CAD build for the part. Positions are in the model's coordinates, mm. A direction names the side the tool comes from. Round coordinates to 2 decimals unless told otherwise and drop trailing zeros. Loops run counter-clockwise (first coordinate to the right, second up) from the corner with the lowest first, then second, coordinate; pieces in that order, holes last.
from build123d import *

# Parameters (mm, degrees)
SKETCH_1_R          = 30
SKETCH_1_R_2        = 1.6
SKETCH_1_R_3        = 13.5
EXTRUDE_1_DEPTH     = 6
SKETCH_2_W          = 8
SKETCH_2_H          = 40
EXTRUDE_2_DEPTH     = 6
SKETCH_3_R          = 1.6
CUT_EXTRUDE_1_DEPTH = 6
SKETCH_4_R          = 3.25
CUT_EXTRUDE_2_DEPTH = 3


with BuildPart() as part:
    # 草图1 → 凸台-拉伸1 (new body)
    with BuildSketch(Plane(origin=(0, 0, 0), x_dir=(1, 0, 0), z_dir=(0, 1, 0))):
        with Locations(Location((15, 90, 0), (0, 0, 270))):
            Circle(SKETCH_1_R)
        with Locations(Location((30.5, 105.5, 0), (0, 0, 270))):
            Circle(SKETCH_1_R_2, mode=Mode.SUBTRACT)
        with Locations(Location((-0.5, 105.5, 0), (0, 0, 270))):
            Circle(SKETCH_1_R_2, mode=Mode.SUBTRACT)
        with Locations(Location((15, 90, 0), (0, 0, 270))):
            Circle(SKETCH_1_R_3, mode=Mode.SUBTRACT)
        with Locations(Location((30.5, 74.5, 0), (0, 0, 270))):
            Circle(SKETCH_1_R_2, mode=Mode.SUBTRACT)
        with Locations(Location((-0.5, 74.5, 0), (0, 0, 270))):
            Circle(SKETCH_1_R_2, mode=Mode.SUBTRACT)
    extrude(amount=EXTRUDE_1_DEPTH)

    # 草图2 → 凸台-拉伸2 (add)
    with BuildSketch(Plane(origin=(0, 6, 0), x_dir=(1, 0, 0), z_dir=(0, 1, 0))):
        with Locations((-11.360679775, 90)):
            Rectangle(SKETCH_2_W, SKETCH_2_H)
    extrude(amount=-EXTRUDE_2_DEPTH)

    # 草图3 → 切除-拉伸1 (cut)
    with BuildSketch(Plane(origin=(0, 6, 0), x_dir=(1, 0, 0), z_dir=(0, 1, 0))):
        with Locations(Location((-11.360679775, 105, 0), (0, 0, 270))):
            Circle(SKETCH_3_R)
        with Locations(Location((-11.360679775, 95, 0), (0, 0, 270))):
            Circle(SKETCH_3_R)
        with Locations(Location((-11.360679775, 85, 0), (0, 0, 270))):
            Circle(SKETCH_3_R)
        with Locations(Location((-11.360679775, 75, 0), (0, 0, 270))):
            Circle(SKETCH_3_R)
    extrude(amount=-CUT_EXTRUDE_1_DEPTH, mode=Mode.SUBTRACT)

    # 草图4 → 切除-拉伸2 (cut)
    with BuildSketch(Plane(origin=(0, 6, 0), x_dir=(1, 0, 0), z_dir=(0, 1, 0))):
        with Locations(Location((-11.360679775, 105, 0), (0, 0, 270))):
            Circle(SKETCH_4_R)
        with Locations(Location((-11.360679775, 95, 0), (0, 0, 270))):
            Circle(SKETCH_4_R)
        with Locations(Location((-11.360679775, 85, 0), (0, 0, 270))):
            Circle(SKETCH_4_R)
        with Locations(Location((-11.360679775, 75, 0), (0, 0, 270))):
            Circle(SKETCH_4_R)
    extrude(amount=-CUT_EXTRUDE_2_DEPTH, mode=Mode.SUBTRACT)


solid = part.part
Item 1: Cut at D-D (z = -105). List the corners of the cut face in (x, y), plus the area to 3 significant figures.
Verdict:
outline: (-15.36, 0) - (-12.96, 0) - (-12.96, 3) - (-14.61, 3) - (-14.61, 6) - (-15.36, 6) - close; (-9.76, 0) - (-2.02, 0) - (-2.02, 6) - (-8.11, 6) - (-8.11, 3) - (-9.76, 3) - close; (1.02, 0) - (28.98, 0) - (28.98, 6) - (1.02, 6) - close; (32.02, 0) - (40.98, 0) - (40.98, 6) - (32.02, 6) - close
area: 272 mm2
Item 2: Wall check: L1, parallel to X at y = 4.4, z = -105.5; L2, parallel to Z at x = -10.5, y = 2.95; L3, parallel to X at y = 5.55, z = -78. Give the ranges that are in metal, low to high.
Verdict:
L1: x = -15.36 to -14.57, -8.15 to -2.1, 1.1 to 28.9, 32.1 to 40.69
L2: z = -110 to -106.35, -103.65 to -96.35, -93.65 to -86.35, -83.65 to -76.35, -73.65 to -70
L3: x = -15.36 to -12.61, -10.11 to 8.82, 21.18 to 42.5
Item 3: Cut at B-B (z = -74.5). List the corners of the cut face in (x, y), plus the area to 3 significant figures.
Verdict:
outline: (-15.36, 0) - (-12.88, 0) - (-12.88, 3) - (-14.57, 3) - (-14.57, 6) - (-15.36, 6) - close; (-9.84, 0) - (-2.1, 0) - (-2.1, 6) - (-8.15, 6) - (-8.15, 3) - (-9.84, 3) - close; (1.1, 0) - (28.9, 0) - (28.9, 6) - (1.1, 6) - close; (32.1, 0) - (40.69, 0) - (40.69, 6) - (32.1, 6) - close
area: 269 mm2
Item 4: Cut at A-A (z = -90). List the corners of the cut face in (x, y), plus the area to 3 significant figures.
Verdict:
outline: (-15.36, 0) - (1.5, 0) - (1.5, 6) - (-15.36, 6) - close; (28.5, 0) - (45, 0) - (45, 6) - (28.5, 6) - close
area: 200 mm2
Item 5: 3-axis set-ups, long thin cutter, end or side, ignore diameter. For faces 4 (the flat face through (-11, 3, -110)), 5 (the flat face through (-11, 3, -70)), 6 (the cylindrical face through (-11.218, 4.521, -108.247)), 7 (the flat face through (28, 6, -84)), 8 (the flat face through (-15.361, 3, -90)): which of +Z, -Z, +X, -X, +Y, -Y reach the whole face in a straight line?
Verdict:
face 4: -Z, -X, +Y, -Y
face 5: +Z, -X, +Y, -Y
face 6: +Y
face 7: +Z, -Z, +X, -X, +Y
face 8: +Z, -Z, -X, +Y, -Y
Item 6: Mould opens along X. For faces 1 (the flat face through (1, 0, -90)), 2 (the flat face through (-13, 3, -104)), 3 (the cylindrical face through (44.983, 2.958, -88.987)) say: released by +X, released by -X, zero draft, split by the parting line, or undercut.
Verdict:
face 1: zero draft
face 2: undercut
face 3: split by the parting line
Item 7: Cut at C-C (y = 0.85). State how many separate pieces and enclosed holes the cut face has, plus the area to 3 significant figures.
Verdict:
separate pieces: 1
enclosed holes: 9
area: 2,300 mm2
Item 8: Flat gauge pins, fed straight in: P1, Ø1.8, axis at x = -12, y = 3, coming from the -Z side; P2, Ø2, axis at x = 24, z = -83.5, coming from the +Y side; P3, Ø2, axis at x = -12.5, z = -103.5, coming from the +Y side; P4, Ø3, axis at y = 1, z = -91, coming from the +X side. Where does each tip first touch, or does it go through?
Verdict:
P1: stops at z = -110
P2: passes through
P3: stops at y = 3
P4: stops at x = 45
